Build history of the part. All positions in model axes, mm. A direction names the side the tool comes from. Give positions to 0.01 mm unless a question says otherwise; leave off trailing zeros. Order: outer loops, then holes, each group sorted by start corner. A loop starts at its lowest first (then second) coordinate and runs counter-clockwise, first axis right, second up. Notation, with made-up numbers: M -38,58 L 16,58 A29 cw 16,96 Z; hole C -10.75,57.25 d1. An arc over 180 degrees is marked long. One line per item, written item: value.
from build123d import *

# Parameters (mm, degrees)
SKETCH1_R               = 14.224
BOSS_EXTRUDE1_DEPTH     = 38.1
F_1_4_CLEARANCE_HOLE1_D = 6.7564
SKETCH4_R               = 16.637181665
SKETCH4_R_2             = 5.08
SKETCH4_R_3             = 1.7
BOSS_EXTRUDE2_DEPTH     = 3
FILLET1_R               = 7.62
CHAMFER1_SIZE           = 1.27


with BuildPart() as part:
    # Sketch1 → Boss-Extrude1 (new body)
    with BuildSketch(Plane.XY):
        with BuildLine():
            Line((-34.29, 0), (34.29, 0))
            Line((34.29, 0), (34.29, 5.08))
            Line((34.29, 5.08), (19.05, 5.08))
            ThreePointArc((19.05, 5.08), (18.151974388, 5.451974388), (17.78, 6.35))
            Line((17.78, 6.35), (17.78, 20.32))
            Line((17.78, 20.32), (17.78, 25.4))
            ThreePointArc((17.78, 25.4), (14.060256121, 34.380256121), (5.08, 38.1))
            Line((5.08, 38.1), (-5.08, 38.1))
            ThreePointArc((-5.08, 38.1), (-14.060256121, 34.380256121), (-17.78, 25.4))
            Line((-17.78, 25.4), (-17.78, 20.32))
            Line((-17.78, 20.32), (-17.78, 6.35))
            ThreePointArc((-17.78, 6.35), (-18.151974388, 5.451974388), (-19.05, 5.08))
            Line((-19.05, 5.08), (-34.29, 5.08))
            Line((-34.29, 5.08), (-34.29, 0))
        make_face()
        with Locations(Location((0, 20.32, 0), (0, 0, 180))):
            Circle(SKETCH1_R, mode=Mode.SUBTRACT)
    extrude(amount=BOSS_EXTRUDE1_DEPTH)

    # 1/4 Clearance Hole1 (through all)
    with Locations(Plane(origin=(0, 5.08, 0), x_dir=(1, 0, 0), z_dir=(0, 1, 0))):
        with Locations((-25.4, -6.35), (25.4, -31.75), (-25.4, -31.75), (25.4, -6.35)):
            Hole(F_1_4_CLEARANCE_HOLE1_D / 2)

    # Sketch4 → Boss-Extrude2 (add)
    with BuildSketch(Plane.XY.offset(38.1)):
        with Locations((0, 20.32)):
            Circle(SKETCH4_R)
        with Locations((0, 20.32)):
            Circle(SKETCH4_R_2, mode=Mode.SUBTRACT)
        with Locations((8.5, 20.32)):
            Circle(SKETCH4_R_3, mode=Mode.SUBTRACT)
        with Locations((-8.5, 20.32)):
            Circle(SKETCH4_R_3, mode=Mode.SUBTRACT)
    extrude(amount=-BOSS_EXTRUDE2_DEPTH)

    # Fillet1
    fillet1_edges = [part.edges().sort_by_distance(p)[0] for p in [
        (-34.29, 2.54, 0),
        (34.29, 2.54, 0),
        (34.29, 2.54, 38.1),
        (-34.29, 2.54, 38.1),
    ]]
    fillet(fillet1_edges, radius=FILLET1_R)

    # Chamfer1
    chamfer1_edges = [part.edges().sort_by_distance(p)[0] for p in [
        (14.224, 20.32, 0),
    ]]
    chamfer(chamfer1_edges, length=CHAMFER1_SIZE)


solid = part.part
1) Mould opens along Z. For faces 5 (the face through (-32.117, 2.504, 2.291)), 6 (the face through (-22.025, 2.504, 6.201)), 7 (the face through (0, 38.1, 19)) say: released by +Z, released by -Z, zero draft, split by the parting line, or undercut.
Check values:
face 5: released by -Z
face 6: undercut
face 7: zero draft
2) Pin check, flat tips, straight feed: pin 1 (7.5 mm diameter, centred on x = 24.5, z = 27.5, fed in from +Y); pin 2 (9.5 mm diameter, centred on y = 12, z = 16.5, fed in from -X); pin 3 (4.5 mm diameter, centred on x = 8.5, y = 20.32, fed in from -Z). Stop position of each tip, or through.
Check values:
pin 1: y = 5.08
pin 2: x = -17.78
pin 3: z = 35.1
3) Drill centre lines: probe 1 along Z at (x, y) = (25.4, 1.95); probe 2 along X at (y, z) = (20.5, 9.5); probe 3 along Y at (x, z) = (0, 37). Where is each one in solid material? Low to high. Write a range as from..to.
Check values:
probe 1: 0..2.97, 9.73..28.37, 35.13..38.1
probe 2: -17.78..-14.22, 14.22..17.78
probe 3: 0..15.24, 25.4..38.1
4) Saw through at A-A, the plane y = 20.32. Write the cut outline in (x, z).
Check values:
outline: M -17.78,0 L -15.49,0 L -14.22,1.27 L -14.22,35.1 L -10.2,35.1 L -10.2,38.1 L -17.78,38.1 Z; M -6.8,35.1 L -5.08,35.1 L -5.08,38.1 L -6.8,38.1 Z; M 5.08,35.1 L 6.8,35.1 L 6.8,38.1 L 5.08,38.1 Z; M 10.2,35.1 L 14.22,35.1 L 14.22,1.27 L 15.49,0 L 17.78,0 L 17.78,38.1 L 10.2,38.1 Z
5) Saw through at D-D, the plane z = 26.5. Write the cut outline in (x, y).
Check values:
outline: M -34.29,0 L 34.29,0 L 34.29,5.08 L 19.05,5.08 A1.27 cw 17.78,6.35 L 17.78,25.4 A12.7 ccw 5.08,38.1 L -5.08,38.1 A12.7 ccw -17.78,25.4 L -17.78,6.35 A1.27 cw -19.05,5.08 L -34.29,5.08 Z; hole C 0,20.32 d28.45
6) Tool access for faces 1 (the face through (-17.78, 16, 19)), 2 (the face through (0, 0, 19)), 3 (the face through (-6.56, 32.94, 17.95)), 4 (the face through (17.78, 16, 19)): list every direction of +Z, -Z, +X, -X, +Y, -Y with a clear straight run to the whole face (end or side of a thin tool).
Check values:
face 1: +Z, -Z, -X, +Y
face 2: +Z, -Z, +X, -X, -Y
face 3: -Z
face 4: +Z, -Z, +X, +Y
7) Saw through at B-B, the plane z = 6.35. Write the cut outline in (x, y), then the cut area to 3 significant figures.
Check values:
outline: M -34.18,0 L -28.78,0 L -28.78,5.08 L -34.18,5.08 Z; M -22.02,0 L 22.02,0 L 22.02,5.08 L 19.05,5.08 A1.27 cw 17.78,6.35 L 17.78,25.4 A12.7 ccw 5.08,38.1 L -5.08,38.1 A12.7 ccw -17.78,25.4 L -17.78,6.35 A1.27 cw -19.05,5.08 L -22.02,5.08 Z; M 28.78,0 L 34.18,0 L 34.18,5.08 L 28.78,5.08 Z; hole C 0,20.32 d28.45
area: 749 mm^2
8) Saw through at C-C, the plane x = 0. Write the cut outline in (y, z).
Check values:
outline: M 0,0 L 4.83,0 L 6.1,1.27 L 6.1,35.1 L 15.24,35.1 L 15.24,38.1 L 0,38.1 Z; M 25.4,35.1 L 34.54,35.1 L 34.54,1.27 L 35.81,0 L 38.1,0 L 38.1,38.1 L 25.4,38.1 Z
